Autodesk Inventor part; units mm, degrees
ref_plane "YZ Plane" through (0, 0, 0) normal (1, 0, 0) x (0, 1, 0)
ref_plane "XZ Plane" through (0, 0, 0) normal (0, 1, 0) x (-1, 0, 0)
ref_plane "XY Plane" through (0, 0, 0) normal (0, 0, 1) x (1, 0, 0)
sketch "Sketch1" plane through (0, 0, 0) normal (0, 0, 1) x (1, 0, 0)
  line L0 (0, 0) -> (25.4, 0)
  line L1 (25.4, 0) -> (25.4, 6.35)
  line L2 (25.4, 6.35) -> (0, 6.35)
  line L3 (0, 6.35) -> (0, 0)
  line L4 (0, 0) -> (6.35, 0)
  line L5 (6.35, 0) -> (6.35, 25.4)
  line L6 (6.35, 25.4) -> (0, 25.4)
  line L7 (0, 25.4) -> (0, 0)
  dimension "d0" = 25.4
  dimension "d1" = 6.35
  dimension "d2" = 6.35
  dimension "d3" = 25.4
extrude "Extrusion1" add sketch "Sketch1" along normal blind 76.2
sketch "Sketch2" plane through (6.35, 6.35, 0) normal (0, 1, 0) x (1, 0, 0)
  line L0 (-6.35, 0) -> (19.05, 0)
  line L1 (19.05, 0) -> (0, 0)
  line L2 (9.525, 0) -> (9.525, -76.2)
  line L3 (-6.35, -76.2) -> (19.05, -76.2)
  line L4 (9.525, 0) -> (9.525, -12.7)
  line L5 (9.525, -76.2) -> (9.525, -63.5)
  circle A0 centre (9.525, -63.5) radius 2.54
  circle A1 centre (9.525, -12.7) radius 2.54
  dimension "d6" = 19.05
  dimension "d7" = 12.7
  dimension "d8" = 12.7
  dimension "d9" = 5.08
  dimension "d10" = 5.08
extrude "Extrusion2" cut sketch "Sketch2" against normal blind 25.4
sketch "Sketch3" plane through (6.35, 6.35, 0) normal (1, 0, 0) x (0, 0, -1)
  line L0 (0, 0) -> (0, 19.05)
  line L1 (0, 0) -> (0, 19.05)
  line L2 (0, 19.05) -> (0, 9.525)
  line L3 (0, 9.525) -> (-76.2, 9.525)
  line L4 (-76.2, 19.05) -> (-76.2, -6.35)
  line L5 (-76.2, 9.525) -> (-63.5, 9.525)
  line L6 (0, 9.525) -> (-12.7, 9.525)
  circle A0 centre (-63.5, 9.525) radius 2.54
  circle A1 centre (-12.7, 9.525) radius 2.54
  point P0 (0, -6.35)
  dimension "d13" = 12.7
  dimension "d14" = 12.7
  dimension "d15" = 5.08
extrude "Extrusion3" cut sketch "Sketch3" against normal blind 25.4
properties part number "Beefy L" material "Aluminum 6061"
Input: part model. Units: mm. Frame: model coordinates. Coordinates: 2 decimals unless noted, no trailing zeros. Loops run counter-clockwise (first coordinate to the right, second up) from the corner with the lowest first, then second, coordinate; pieces in that order, holes last.
Q1. Cut plane B-B (y = 14.5). Output: boundary loops of the cut face in (x, z).
Q2. Cut plane A-A (z = 12.7). Output: boundary loops of the cut face in (x, y) (3 decimals), then the cut area to 3 significant figures.
Q3. Material intervals for line 1 (Y direction, x = 3.5, z = 12.7) (3 decimals); line 2 (X direction, y = 2, z = 12.5); line 3 (X direction, y = 22.25, z = 37), sorted ascending.
Q4. Cut plane C-C (x = 16.25). Output: boundary loops of the cut face in (y, z), then the cut area to 3 significant figures.
Q5. Cut plane D-D (y = 1.5). Output: boundary loops of the cut face in (x, z) (3 decimals).
Q6. Contact query for flat-ended pins moving along their axis: pin 1 (4 mm diameter, centred on x = 9.5, z = 59, fed in from +Y); pin 2 (8 mm diameter, centred on y = 15.875, z = 12.7, fed in from +X); pin 3 (3 mm diameter, centred on y = 15.875, z = 63.5, fed in from -X). Output: stop coordinate, or through.
Q7. Draft query along Y for faces 1 (the face through (6.35, 16, 38)), 2 (the face through (3.219, 14.329, 65.516)), 3 (the face through (16, 6.35, 38)). Return one class per face: +Y half, -Y half, draft (parallel to the pull), parting line (faces both ways), or undercut.
Working result:
1. outline: (0, 0) - (6.35, 0) - (6.35, 10.56) - (0, 10.56) - close; (0, 14.84) - (6.35, 14.84) - (6.35, 61.36) - (0, 61.36) - close; (0, 65.64) - (6.35, 65.64) - (6.35, 76.2) - (0, 76.2) - close
2. outline: (0, 0) - (13.335, 0) - (13.335, 6.35) - (6.35, 6.35) - (6.35, 13.335) - (0, 13.335) - close; (0, 18.415) - (6.35, 18.415) - (6.35, 25.4) - (0, 25.4) - close; (18.415, 0) - (25.4, 0) - (25.4, 6.35) - (18.415, 6.35) - close
2. area: 218 mm2
3. line 1: y = 0 to 13.335, 18.415 to 25.4
3. line 2: x = 0 to 13.34, 18.41 to 25.4
3. line 3: x = 0 to 6.35
4. outline: (0, 0) - (6.35, 0) - (6.35, 10.19) - (0, 10.19) - close; (0, 15.21) - (6.35, 15.21) - (6.35, 60.99) - (0, 60.99) - close; (0, 66.01) - (6.35, 66.01) - (6.35, 76.2) - (0, 76.2) - close
4. area: 420 mm2
5. outline: (0, 0) - (25.4, 0) - (25.4, 76.2) - (0, 76.2) - close; hole circle Ø5.08 at (15.875, 12.7); hole circle Ø5.08 at (15.875, 63.5)
6. pin 1: stops at y = 6.35
6. pin 2: stops at x = 6.35
6. pin 3: passes through
7. face 1: draft
7. face 2: undercut
7. face 3: +Y half
